Design review of the part built by this model. Coordinates are the model's own, in mm. Coordinates: 2 decimals unless noted, no trailing zeros. Loops run counter-clockwise (first coordinate to the right, second up) from the corner with the lowest first, then second, coordinate; pieces in that order, holes last. Notation, with made-up numbers: (43.25, 31.5) -> (99.25, 31.5) arc R9 ccw to (99.25, 39.5) -> close; hole circle Ø4 at (63, 43.5). An arc over 180 degrees is marked (long way). Use a Markdown table: item, result. Add a question column.
Q1. Clearance check with flat-ended pins moving along their axes: pin 1 Ø0.9 at (y, z) = (0.5, 1) entering from -X; pin 2 Ø0.9 at (y, z) = (0.5, 1) entering from +X. State where each tip first meets the part, or that it passes through.
Q2. Take a section at C-C on x = -11. Write out the cut boundary in (y, z).
Q3. Take a section at D-D on z = 2.3. Count the separate pieces of the cut face and the enclosed holes in it, plus the area to 3 significant figures.
Q4. Take a section at A-A on y = 53.25. Write out the cut boundary in (x, z), plus the area to 3 significant figures.
Q5. Take a section at B-B on y = 25.25. Write out the cut boundary in (x, z), plus the area to 3 significant figures.
Q6. For probe 1 along Y at (x, z) = (0, 1.4); probe 2 along Y at (x, z) = (9, 1.75); probe 3 along Y at (x, z) = (-11, 1.9), list the stretches that pass through material, from the lowest coordinate up.
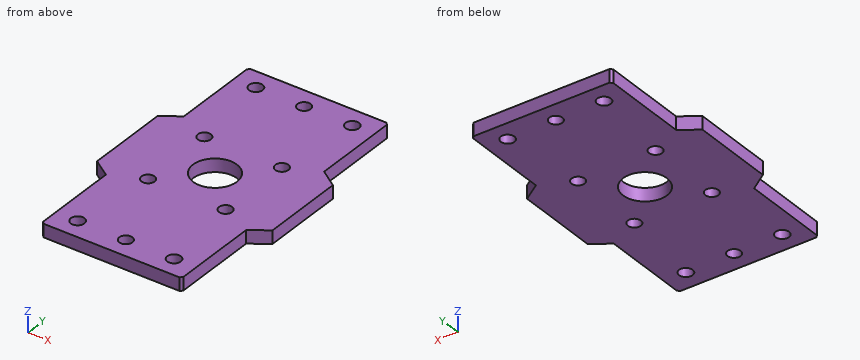
from build123d import *

# Parameters (mm, degrees)
IZIM1_R                      = 1
Y_KSEKLIK_EKSTR_ZYON1_DEPTH  = 3
KES_EKSTR_ZYON1_DEPTH        = 10
Y_KSEKLIK_EKSTR_ZYON2_DEPTH  = 3
IZIM6_R                      = 1.55
Y_KSEKLIK_EKSTR_ZYON4_DEPTH  = 3
IZIM9_W                      = 2.764853826
IZIM9_H                      = 2.899724745
IZIM9_W_2                    = 2.53555673
IZIM9_H_2                    = 2.630505748
Y_KSEKLIK_EKSTR_ZYON5_DEPTH  = 3
IZIM8_R                      = 1.55
Y_KSEKLIK_EKSTR_ZYON6_DEPTH  = 3
IZIM10_R                     = 1.55
KES_EKSTR_ZYON2_DEPTH        = 10
IZIM14_R                     = 1.5
KES_EKSTR_ZYON3_DEPTH        = 10
IZIM15_R                     = 5
KES_EKSTR_ZYON4_DEPTH        = 10
Y_KSEKLIK_EKSTR_ZYON7_DEPTH  = 3
KES_EKSTR_ZYON5_DEPTH        = 3
IZIM23_R                     = 1.55
KES_EKSTR_ZYON6_DEPTH        = 3
IZIM25_R                     = 1.5
KES_EKSTR_ZYON7_DEPTH        = 3
Y_KSEKLIK_EKSTR_ZYON8_DEPTH  = 3
IZIM27_W                     = 26
IZIM27_H                     = 10
Y_KSEKLIK_EKSTR_ZYON9_DEPTH  = 3
IZIM28_W                     = 32
IZIM28_H                     = 10.183470431
KES_EKSTR_ZYON8_DEPTH        = 10
IZIM29_W                     = 21.597894427
IZIM29_H                     = 9.610197834
Y_KSEKLIK_EKSTR_ZYON11_DEPTH = 3
IZIM30_W                     = 32
IZIM30_H                     = 0.75
IZIM30_H_2                   = 0.5
KES_EKSTR_ZYON9_DEPTH        = 10
PAH1_SIZE                    = 0.5


with BuildPart() as part:
    # Çizim1 → Yükseklik-Ekstrüzyon1 (new body)
    # profile 1 of 2: a face of its own
    with BuildSketch(Plane.XY):
        Polygon((7.5, 49.5), (0, 49.5), (0, 46.25495549), (3, 46.25495549), (3.494974747, 46.749930237), (5.494974747, 46.749930237), (8.5, 44.749930237), (8.5, 43.249930237), (8.5, 41.749930237), (5.494974747, 39.749930237), (3.494974747, 39.749930237), (3, 40.244904984), (0, 40.244904984), (0, -51.5), (8.5, -51.5), (13.25, -48.202566926), (13.25, -43.75), (12.5, -43), (12.5, -35), (13.25, -34.25), (13.25, -28.25), (12.5, -27.5), (12.5, -19.5), (13.25, -18.75), (13.25, -12.75), (12.5, -12), (12.5, -4), (14, -2.5), (14, -2), (16, 0), (16, 13), (20, 15.75), (20, 33.5), (20, 34.75), (16, 37.5), (16, 47.5), (12, 51.5), (9.5, 51.5), align=None)
        Polygon((2.624434095, -42.600069763), (3.119408841, -42.105095016), (3.119408841, -36.105095016), (2.624434095, -35.610120269), (2.624434095, -33.610120269), (4.624434095, -30.605095016), (6.124434095, -30.605095016), (7.624434095, -30.605095016), (9.624434095, -33.610120269), (9.624434095, -35.610120269), (9.129459348, -36.105095016), (9.129459348, -42.105095016), (9.624434095, -42.600069763), (9.624434095, -44.600069763), (7.624434095, -47.605095016), (6.124434095, -47.605095016), (4.624434095, -47.605095016), (2.624434095, -44.600069763), align=None, mode=Mode.SUBTRACT)
        Polygon((4.624434095, -7.305095016), (6.124434095, -7.305095016), (7.624434095, -7.305095016), (9.624434095, -10.310120269), (9.624434095, -12.310120269), (9.129459348, -12.805095016), (9.129459348, -18.805095016), (9.624434095, -19.300069763), (9.624434095, -21.300069763), (7.624434095, -24.305095016), (6.124434095, -24.305095016), (4.624434095, -24.305095016), (2.624434095, -21.300069763), (2.624434095, -19.300069763), (3.119408841, -18.805095016), (3.119408841, -12.805095016), (2.624434095, -12.310120269), (2.624434095, -10.310120269), align=None, mode=Mode.SUBTRACT)
        with Locations((11, -0.75)):
            Circle(IZIM1_R, mode=Mode.SUBTRACT)
        with Locations((11, 48.25)):
            Circle(IZIM1_R, mode=Mode.SUBTRACT)
    # profile 2 of 2: a face of its own
    with BuildSketch(Plane.XY):
        Polygon((-9.5, 51.5), (-12, 51.5), (-16, 47.5), (-16, 37.5), (-20, 34.75), (-20, 33.5), (-20, 15.75), (-16, 13), (-16, 0), (-14, -2), (-14, -2.5), (-12.5, -4), (-12.5, -12), (-13.25, -12.75), (-13.25, -18.75), (-12.5, -19.5), (-12.5, -27.5), (-13.25, -28.25), (-13.25, -34.25), (-12.5, -35), (-12.5, -43), (-13.25, -43.75), (-13.25, -48.202566926), (-8.5, -51.5), (0, -51.5), (0, 40.244904984), (-3, 40.244904984), (-3.494974747, 39.749930237), (-5.494974747, 39.749930237), (-8.5, 41.749930237), (-8.5, 43.249930237), (-8.5, 44.749930237), (-5.494974747, 46.749930237), (-3.494974747, 46.749930237), (-3, 46.25495549), (0, 46.25495549), (0, 49.5), (-7.5, 49.5), align=None)
        Polygon((-2.624434095, -35.610120269), (-3.119408841, -36.105095016), (-3.119408841, -42.105095016), (-2.624434095, -42.600069763), (-2.624434095, -44.600069763), (-4.624434095, -47.605095016), (-6.124434095, -47.605095016), (-7.624434095, -47.605095016), (-9.624434095, -44.600069763), (-9.624434095, -42.600069763), (-9.129459348, -42.105095016), (-9.129459348, -36.105095016), (-9.624434095, -35.610120269), (-9.624434095, -33.610120269), (-7.624434095, -30.605095016), (-6.124434095, -30.605095016), (-4.624434095, -30.605095016), (-2.624434095, -33.610120269), align=None, mode=Mode.SUBTRACT)
        with Locations((-11, -0.75)):
            Circle(IZIM1_R, mode=Mode.SUBTRACT)
        Polygon((-3.119408841, -18.805095016), (-2.624434095, -19.300069763), (-2.624434095, -21.300069763), (-4.624434095, -24.305095016), (-6.124434095, -24.305095016), (-7.624434095, -24.305095016), (-9.624434095, -21.300069763), (-9.624434095, -19.300069763), (-9.129459348, -18.805095016), (-9.129459348, -12.805095016), (-9.624434095, -12.310120269), (-9.624434095, -10.310120269), (-7.624434095, -7.305095016), (-6.124434095, -7.305095016), (-4.624434095, -7.305095016), (-2.624434095, -10.310120269), (-2.624434095, -12.310120269), (-3.119408841, -12.805095016), align=None, mode=Mode.SUBTRACT)
        with Locations((-11, 48.25)):
            Circle(IZIM1_R, mode=Mode.SUBTRACT)
    extrude(amount=Y_KSEKLIK_EKSTR_ZYON1_DEPTH)

    # Çizim2 → Kes-Ekstrüzyon1 (cut)
    with BuildSketch(Plane.XY.offset(3)):
        Polygon((-12.5, -4), (12.5, -4), (38.548396408, -28.529419771), (17.359301926, -71.305004234), (-44.147930668, -53.058839542), align=None)
    extrude(amount=-KES_EKSTR_ZYON1_DEPTH, mode=Mode.SUBTRACT)

    # Çizim3 → Yükseklik-Ekstrüzyon2 (add)
    with BuildSketch(Plane.XY.offset(3)):
        Polygon((9.5, 51.5), (-9.5, 51.5), (-7.5, 49.5), (7.5, 49.5), align=None)
    extrude(amount=-Y_KSEKLIK_EKSTR_ZYON2_DEPTH)

    # Çizim6 → Yükseklik-Ekstrüzyon4 (add)
    with BuildSketch(Plane.XY.offset(3)):
        Polygon((-16, 47.5), (-16, 54.5), (-12, 58.5), (12, 58.5), (16, 54.5), (16, 47.5), (12.510789388, 45.937791763), (6.230146787, 48.369008254), (-4.136290194, 49.078113063), (-9.944196255, 45.397521432), align=None)
        with Locations((11, 53.25)):
            Circle(IZIM6_R, mode=Mode.SUBTRACT)
        with Locations((-11, 53.25)):
            Circle(IZIM6_R, mode=Mode.SUBTRACT)
    extrude(amount=-Y_KSEKLIK_EKSTR_ZYON4_DEPTH)

    # Çizim9 → Yükseklik-Ekstrüzyon5 (add)
    with BuildSketch(Plane.XY.offset(3)):
        with Locations((-10.828696241, -0.299998429)):
            Rectangle(IZIM9_W, IZIM9_H)
        with Locations((11.040614903, -0.603719415)):
            Rectangle(IZIM9_W_2, IZIM9_H_2)
    extrude(amount=-Y_KSEKLIK_EKSTR_ZYON5_DEPTH)

    # Çizim8 → Yükseklik-Ekstrüzyon6 (add)
    with BuildSketch(Plane.XY.offset(3)):
        Polygon((-16, 0), (-16, -2), (-12.5, -6), (12.5, -6), (16, -2), (16, 0), (12.001079667, 1.705733335), (6.853090616, -1.163543143), (-3.589444332, -1.163543143), (-11.459943544, 2.530439958), align=None)
        with Locations((-11, -2.75)):
            Circle(IZIM8_R, mode=Mode.SUBTRACT)
        with Locations((11, -2.75)):
            Circle(IZIM8_R, mode=Mode.SUBTRACT)
    extrude(amount=-Y_KSEKLIK_EKSTR_ZYON6_DEPTH)

    # Çizim10 → Kes-Ekstrüzyon2 (cut)
    with BuildSketch(Plane.XY.offset(3)):
        with Locations((-11, -2.75)):
            Circle(IZIM10_R)
        with Locations((11, -2.75)):
            Circle(IZIM10_R)
    extrude(amount=-KES_EKSTR_ZYON2_DEPTH, mode=Mode.SUBTRACT)

    # Çizim14 → Kes-Ekstrüzyon3 (cut)
    with BuildSketch(Plane.XY.offset(3)):
        with Locations((8.838834765, 34.088834765)):
            Circle(IZIM14_R)
        with Locations((-8.838834765, 16.411165235)):
            Circle(IZIM14_R)
        with Locations((8.838834765, 16.411165235)):
            Circle(IZIM14_R)
        with Locations((-8.838834765, 34.088834765)):
            Circle(IZIM14_R)
    extrude(amount=-KES_EKSTR_ZYON3_DEPTH, mode=Mode.SUBTRACT)

    # Çizim15 → Kes-Ekstrüzyon4 (cut)
    with BuildSketch(Plane.XY.offset(3)):
        with Locations((0, 25.25)):
            Circle(IZIM15_R)
    extrude(amount=-KES_EKSTR_ZYON4_DEPTH, mode=Mode.SUBTRACT)

    # Çizim19 → Yükseklik-Ekstrüzyon7 (add)
    with BuildSketch(Plane.XY.offset(3)):
        Polygon((-16, -13), (-12, -17), (12, -17), (16, -13), (16, -2), (-16, -2), align=None)
    extrude(amount=-Y_KSEKLIK_EKSTR_ZYON7_DEPTH)

    # Çizim22 → Kes-Ekstrüzyon5 (cut)
    with BuildSketch(Plane.XY.offset(3)):
        Polygon((3, -7.610667932), (3.494974747, -7.115693185), (5.494974747, -7.115693185), (8.5, -9.115693185), (8.5, -12.115693185), (5.494974747, -14.115693185), (3.494974747, -14.115693185), (3, -13.620718438), (-3, -13.620718438), (-3.494974747, -14.115693185), (-5.494974747, -14.115693185), (-8.5, -12.115693185), (-8.5, -9.115693185), (-5.494974747, -7.115693185), (-3.494974747, -7.115693185), (-3, -7.610667932), align=None)
    extrude(amount=-KES_EKSTR_ZYON5_DEPTH, mode=Mode.SUBTRACT)

    # Çizim23 → Kes-Ekstrüzyon6 (cut)
    with BuildSketch(Plane.XY.offset(3)):
        with Locations((-11, -2.75)):
            Circle(IZIM23_R)
        with Locations((11, -2.75)):
            Circle(IZIM23_R)
    extrude(amount=-KES_EKSTR_ZYON6_DEPTH, mode=Mode.SUBTRACT)

    # Çizim25 → Kes-Ekstrüzyon7 (cut)
    with BuildSketch(Plane.XY.offset(3)):
        with Locations((0, -2.75)):
            Circle(IZIM25_R)
        with Locations((0, 53.25)):
            Circle(IZIM25_R)
    extrude(amount=-KES_EKSTR_ZYON7_DEPTH, mode=Mode.SUBTRACT)

    # Çizim26 → Yükseklik-Ekstrüzyon8 (add)
    with BuildSketch(Plane.XY.offset(3)):
        Polygon((-16, 54.5), (-12, 58.5), (-16, 58.5), align=None)
        Polygon((12, 58.5), (16, 54.5), (16, 58.5), align=None)
    extrude(amount=-Y_KSEKLIK_EKSTR_ZYON8_DEPTH)

    # Çizim27 → Yükseklik-Ekstrüzyon9 (add)
    with BuildSketch(Plane.XY.offset(3)):
        with Locations((-1, -12)):
            Rectangle(IZIM27_W, IZIM27_H)
    extrude(amount=-Y_KSEKLIK_EKSTR_ZYON9_DEPTH)

    # Çizim28 → Kes-Ekstrüzyon8 (cut)
    with BuildSketch(Plane.XY.offset(3)):
        with Locations((0, -12.841735215)):
            Rectangle(IZIM28_W, IZIM28_H)
    extrude(amount=-KES_EKSTR_ZYON8_DEPTH, mode=Mode.SUBTRACT)

    # Çizim29 → Yükseklik-Ekstrüzyon11 (add)
    with BuildSketch(Plane.XY.offset(3)):
        with Locations((0.687303888, 43.184879182)):
            Rectangle(IZIM29_W, IZIM29_H)
    extrude(amount=-Y_KSEKLIK_EKSTR_ZYON11_DEPTH)

    # Çizim30 → Kes-Ekstrüzyon9 (cut)
    with BuildSketch(Plane.XY.offset(3)):
        with Locations((0, 58.125)):
            Rectangle(IZIM30_W, IZIM30_H)
        with Locations((0, -7.5)):
            Rectangle(IZIM30_W, IZIM30_H_2)
    extrude(amount=-KES_EKSTR_ZYON9_DEPTH, mode=Mode.SUBTRACT)

    # Pah1
    pah1_edges = [part.edges().sort_by_distance(p)[0] for p in [
        (16, 57.75, 1.5),
        (-16, 57.75, 1.5),
        (-16, -7.25, 1.5),
        (16, -7.25, 1.5),
    ]]
    chamfer(pah1_edges, length=PAH1_SIZE)


solid = part.part
Answer list:
| question | item | result |
|---|---|---|
| 1 | pin 1 | x = -16 |
| 1 | pin 2 | x = 16 |
| 2 | outline | (-7.25, 0) -> (-4.3, 0) -> (-4.3, 3) -> (-7.25, 3) -> close; (-1.2, 0) -> (51.7, 0) -> (51.7, 3) -> (-1.2, 3) -> close; (54.8, 0) -> (57.75, 0) -> (57.75, 3) -> (54.8, 3) -> close |
| 3 | separate pieces | 1 |
| 3 | enclosed holes | 11 |
| 3 | area | 2,100 mm² |
| 4 | outline | (-16, 0) -> (-12.55, 0) -> (-12.55, 3) -> (-16, 3) -> close; (-9.45, 0) -> (-1.5, 0) -> (-1.5, 3) -> (-9.45, 3) -> close; (1.5, 0) -> (9.45, 0) -> (9.45, 3) -> (1.5, 3) -> close; (12.55, 0) -> (16, 0) -> (16, 3) -> (12.55, 3) -> close |
| 4 | area | 68.4 mm² |
| 5 | outline | (-20, 0) -> (-5, 0) -> (-5, 3) -> (-20, 3) -> close; (5, 0) -> (20, 0) -> (20, 3) -> (5, 3) -> close |
| 5 | area | 90.0 mm² |
| 6 | probe 1 | -7.25 to -4.25, -1.25 to 20.25, 30.25 to 51.75, 54.75 to 57.75 |
| 6 | probe 2 | -7.25 to 14.92, 17.9 to 32.6, 35.58 to 57.75 |
| 6 | probe 3 | -7.25 to -4.3, -1.2 to 51.7, 54.8 to 57.75 |
